The figure shows three views and two pictorial views of one solid part (mm, origin at its lowest corner). Answer the questions. A direction names the side the tool comes from. Round coordinates to 2 decimals unless told otherwise and drop trailing zeros. Order: outer loops, then holes, each group sorted by start corner. A loop starts at its lowest first (then second) coordinate and runs counter-clockwise, first axis right, second up. Notation, with made-up numbers: (-7, 8) - (51, 8) arc R26 ccw to (51, 32) - close; hole circle Ø8 at (-6, 12). An arc over 180 degrees is marked (long way). One line per item, written item: value. Start each with the question number.
1. Section A-A, the plane y = 55.5 is taken. Give the vertices of the cut face in (x, z).
2. Straight lines are drawn through the part: line 1 (Y direction, x = 241.5, z = 77); line 2 (Z direction, x = 208.5, y = 15.5); line 3 (Z direction, x = 363.5, y = 9) (1 decimal). For each, find the intervals that lie inside material, in ascending order.
3. Section D-D, the plane x = 56 is taken. Give the vertices of the cut face in (y, z).
4. A tool of negligible diameter and unlimited length cuts with its end or side. For the marked faces 1, 2 and 3, from which of +Z, -Z, +X, -X, +Y, -Y can it reach the whole face along a straight path? Write none if from no direction.
5. Flat-ended cylindrical pins translate along their axes: P1, Ø6, axis at x = 264, z = 35.5, coming from the +Y side (1 decimal); P2, Ø12, axis at x = 115.5, z = 24, coming from the -Y side; P3, Ø4.5, axis at x = 242, z = 27, coming from the +Y side; P4, Ø9.5, axis at x = 334.74, z = 64.22, coming from the +Y side. Find the tip coordinate at first contact, or state that the pin passes through.
6. Section B-B, the plane x = 200 is taken. Give the vertices of the cut face in (y, z).
7. Section C-C, the plane z = 7.5 is taken. Give the vertices of the cut face in (x, y).
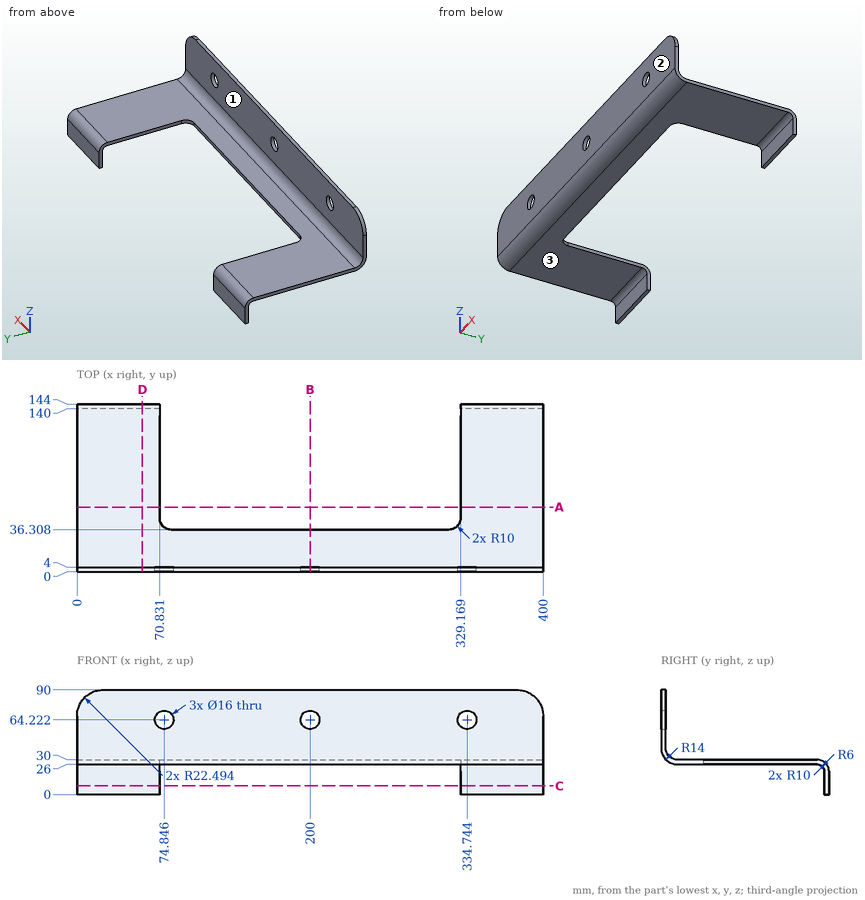
Answer list:
1. outline: (0, 26) - (70.83, 26) - (70.83, 30) - (0, 30) - close; (329.17, 26) - (400, 26) - (400, 30) - (329.17, 30) - close
2. line 1: y = 0 to 4
2. line 2: z = 26 to 30
2. line 3: z = 26.9 to 31.3
3. outline: (0, 40) arc R14 ccw to (14, 26) - (134, 26) arc R6 cw to (140, 20) - (140, 0) - (144, 0) - (144, 20) arc R10 ccw to (134, 30) - (14, 30) arc R10 cw to (4, 40) - (4, 90) - (0, 90) - close
4. face 1: +Z, +X, -X, +Y
4. face 2: +Z, -Z, +X, -X, -Y
4. face 3: -Z, +X, -X, -Y
5. P1: stops at y = 7.4
5. P2: stops at y = 4.2
5. P3: stops at y = 36.31
5. P4: passes through
6. outline: (0, 40) arc R14 ccw to (14, 26) - (36.31, 26) - (36.31, 30) - (14, 30) arc R10 cw to (4, 40) - (4, 56.22) - (0, 56.22) - close; (0, 72.22) - (4, 72.22) - (4, 90) - (0, 90) - close
7. outline: (0, 140) - (70.83, 140) - (70.83, 144) - (0, 144) - close; (329.17, 140) - (400, 140) - (400, 144) - (329.17, 144) - close
